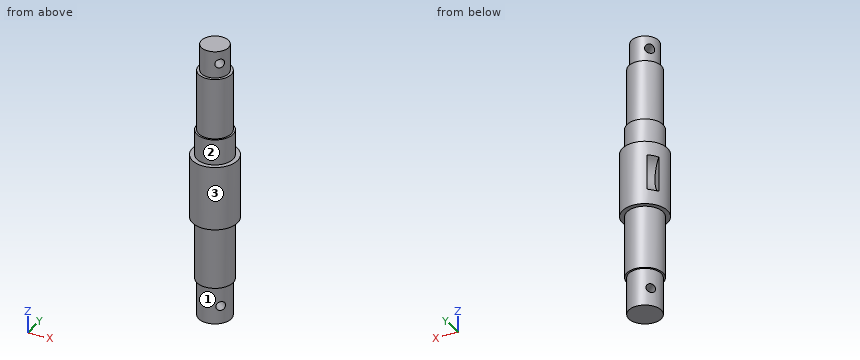
Autodesk Inventor part; units mm, degrees
ref_plane "Work Plane2" through (0, 0, 0) normal (-0.6701796, -0.7421989, 0) x (0, 0, 1)
ref_plane "YZ Plane" through (0, 0, 0) normal (1, 0, 0) x (0, 1, 0)
ref_plane "XZ Plane" through (0, 0, 0) normal (0, 1, 0) x (-1, 0, 0)
sketch "Sketch1" plane through (0, 0, 0) normal (0, 1, 0) x (-1, 0, 0)
  line L0 (0, 0) -> (0, -155)
  line L1 (0, -155) -> (9, -155)
  line L2 (9, -155) -> (9, -134)
  line L3 (9, -134) -> (10, -134)
  line L4 (10, -134) -> (10, -99)
  line L5 (10, -99) -> (12.5, -99)
  line L6 (12.5, -99) -> (12.5, -63.3)
  line L7 (12.5, -63.3) -> (10, -63.3)
  line L8 (10, -63.3) -> (10, -49)
  line L9 (10, -49) -> (9, -49)
  line L10 (9, -49) -> (9, -15)
  line L11 (9, -15) -> (7.5, -15)
  line L12 (7.5, -15) -> (7.5, 0)
  line L13 (7.5, 0) -> (0, 0)
  dimension "d1" = 155
  dimension "d2" = 9
  dimension "d3" = 21
  dimension "d4" = 1
  dimension "d5" = 35
  dimension "d6" = 2.5
  dimension "d7" = 35.7
  dimension "d8" = 2.5
  dimension "d9" = 14.3
  dimension "d10" = 1
  dimension "d11" = 34
  dimension "d12" = 1.5
  dimension "d13" = 15
revolve "Revolution1" add sketch "Sketch1" angle 360 about axis through (0, 0, 0) along (0, 0, -1)
sketch "Sketch2" plane through (0, 0, -155) normal (0, 0, -1) x (-1, 0, 0)
  circle A0 centre (0, 0) radius 9
  circle A1 centre (0, 0) radius 7.5
  point P0 (6.6798, 6.0316)
ref_plane "Work Plane1" through (-6.6798, 6.0316, -155) normal (-0.7421989, 0.6701796, 0) x (-0.6701796, -0.7421989, 0)
sketch "Sketch3" plane through (-6.6798, 6.0316, -155) normal (-0.7421989, 0.6701796, 0) x (-0.6701796, -0.7421989, 0)
  line L0 (-9, 0) -> (9, 0)
  circle A0 centre (0, 10) radius 2.5
  point P0 (0, 155)
  dimension "d17" = 5
  dimension "d18" = 10
extrude "Extrusion1" cut sketch "Sketch3" against normal through all
ref_plane "Work Plane2" through (0, 0, 0) normal (-0.6701796, -0.7421989, 0) x (0, 0, 1)
sketch "Sketch4" plane through (0, 0, 0) normal (-0.6701796, -0.7421989, 0) x (0, 0, 1)
  line L0 (-99, 12.5) -> (-99, -12.5)
  line L1 (-57, 0) -> (-57, 17.3) construction
  line L2 (-81, 17.2999) -> (-81, -8.0858) construction
  line L3 (-57, 17.3) -> (-99, 17.3) construction
  arc A0 (-90.8975, 12.5) -> (-71.1025, 12.5) centre (-81, 17.2999) ccw
  line L4 (-63.3, 12.5) -> (-99, 12.5)
  point P0 (0, 0)
  dimension "d22" = 17.3
  dimension "d24" = 18
  dimension "d25" = 24
  dimension "d27" = 11
  dimension "d28" = 19.795
extrude "Extrusion2" cut sketch "Sketch4" along normal mid plane 6
sketch "Sketch5" plane through (0, 0, 0) normal (-0.6701796, -0.7421989, 0) x (0, 0, 1)
  line L0 (-15, 9) -> (-15, -9)
  line L1 (-15, 9) -> (-7, 9) construction
  line L2 (-15, 9) -> (-49, 9) construction
  line L3 (-7, 9) -> (-7, 7.5) construction
  line L4 (0, 7.5) -> (-15, 7.5) construction
  line L5 (-7, 7.5) -> (-9.65, 7.5) construction
  line L6 (-7, 7.5) -> (-7, -7.5) construction
  line L7 (0, -7.5) -> (-15, -7.5) construction
  line L8 (-7, -7.5) -> (-9.5, -7.5) construction
  line L9 (-9.5, -7.5) -> (-9.65, 7.5) construction
  line L10 (-7, 7.5) -> (-9.65, 7.5)
  line L11 (-9.5, -7.5) -> (-7, -7.5)
  line L12 (-7, 7.5) -> (-7, -7.5)
  line L13 (-9.5, -7.5) -> (-9.65, 7.5)
  point P0 (0, 0)
  dimension "d31" = 8
  dimension "d41" = 2.65
  dimension "d42" = 2.5
revolve "Revolution2" cut sketch "Sketch5" angle 360 about axis through (-5.5665, 5.0263, -7) along (0.7421989, -0.6701796, 0)
properties part number "laborator2 final"
Design review of the part built by this model. Coordinates are the model's own, in mm. Face numbers are marked on the shaded views. A direction names the side the tool comes from. Round coordinates to 2 decimals unless told otherwise and drop trailing zeros. Write each loop counter-clockwise with the first axis right and the second up, starting at its lowest first coordinate (ties: lowest second). Pieces come first, ordered by that corner, then holes. Notation, with made-up numbers: (21.25, 67.25) -> (53.25, 67.25) arc R22 ccw to (53.25, 92.25) -> close; hole circle Ø4 at (-14.5, -37). An arc over 180 degrees is marked (long way). Write item = value, one per line. Start each with the question number.
1) Tool access review of the marked faces 1, 2 and 3: name each direction out of +Z, -Z, +X, -X, +Y, -Y from which nothing blocks a thin tool from reaching the whole face with its end or side.
2) Take a section at B-B, the plane x = -0.75. Count the separate pieces of the cut face and the enclosed holes in it, plus the area to 3 significant figures.
3) Take a section at A-A, the plane z = -24. State the section outline as (x, y) points.
4) Wall thickness on probe 1 along Z at (x, y) = (9.75, -7.25); probe 2 along Y at (x, z) = (-3, -81); probe 3 along Z at (x, y) = (0, -0.5): over which ranges is each line inside the solid? List them lowest first. Write a range as from..to.
5) Clearance check with flat-ended pins moving along their axes: pin 1 (2 mm diameter, centred on y = -2.5, z = -36.5, fed in from +X); pin 2 (1.5 mm diameter, centred on x = 5, z = -16.5, fed in from -Y); pin 3 (5 mm diameter, centred on x = 10, y = -8.5, fed in from +Z). State where each tip first meets the part, or that it passes through.
Results list:
q1.face_1 = -Z
q1.face_2 = +Z
q1.face_3 = +Z, -Z
q2.separate_pieces = 1
q2.enclosed_holes = 2
q2.area = 3,030 mm²
q3.outline = circle Ø18 at (0, 0)
q4.probe_1 = -99..-63.3
q4.probe_2 = -12.13..6.08, 6.75..12.13
q4.probe_3 = -155..-147.47, -142.53..-9.54, -4.46..0
q5.pin_1 = 8.87
q5.pin_2 = -7.93
q5.pin_3 = -63.3
